Geometry: final body of the model. Coordinates: model frame, mm. Face numbers are marked on the shaded views. A direction names the side the tool comes from. Give positions to 0.01 mm unless a question says otherwise; leave off trailing zeros. Write each loop counter-clockwise with the first axis right and the second up, starting at its lowest first coordinate (ties: lowest second). Pieces come first, ordered by that corner, then holes. Notation, with made-up numbers: (-33.75, 83) -> (-5.75, 83) arc R17 cw to (-5.75, 96) -> close; hole circle Ø2 at (87, 58). An arc over 180 degrees is marked (long way). Answer in a Markdown table with one row per item. Add a question column.
Item 1: First-contact query: P1, Ø1.5, axis at x = 14, z = -6.5, coming from the -Y side; P2, Ø2.5, axis at y = 1.5, z = -5, coming from the -X side; P3, Ø2, axis at x = 4, z = 9, coming from the -Y side. Flat tips, straight axial feed; report the tip coordinate or a pass-through.
Item 2: Material intervals for probe 1 along Z at (x, y) = (0, 8.6); probe 2 along Z at (x, y) = (-10, 9.75); probe 3 along X at (y, z) = (1, -1), sorted ascending. Write a range as from..to.
Item 3: Section query D-D on z = 4. Output: boundary loops of the cut face in (x, y).
Item 4: Draft query along X for the marked faces 1, 2, 3 and 4. Return one class per face: +X half, -X half, draft (parallel to the pull), parting line (faces both ways), or undercut.
Item 5: Section query C-C on x = 0. Output: boundary loops of the cut face in (y, z).
Item 6: Section query B-B on y = 4. Output: boundary loops of the cut face in (x, z).
Item 7: Access query for the marked faces 5, 6 and 7. Directions: +Z, -Z, +X, -X, +Y, -Y. A direction counts if a zero-diameter tool reaches every point of the face in a straight line with its end or side. Return the directions, or none.
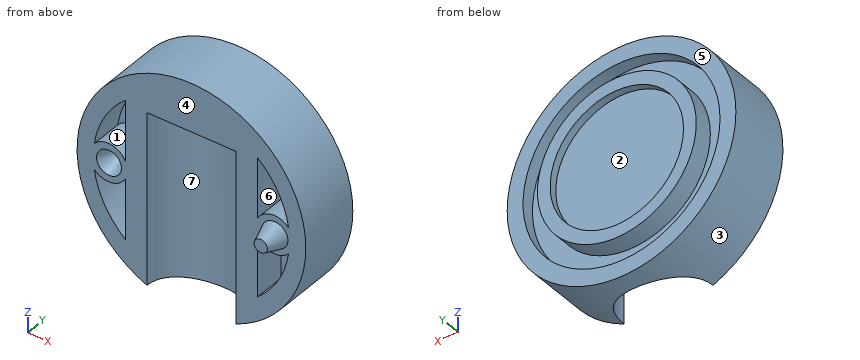
```python
from build123d import *

# Parameters (mm, degrees)
F0_R      = 18
F1_DEPTH  = 10
F2_R      = 15.5
F3_DEPTH  = 2
F5_DEPTH  = 5
F6_R      = 3
F6_R_2    = 1.5
F7_DEPTH  = 5
F8_R      = 12.5
F9_DEPTH  = 3
F10_R     = 10.5
F11_DEPTH = 1.2
F16_W     = 7
F16_H     = 30.015691
F17_ANGLE = -180


with BuildPart() as f1:
    # F0 (on Front) → F1 (new body)
    with BuildSketch(Plane.XZ):
        Circle(F0_R)
    extrude(amount=-F1_DEPTH)

    # F2 (on face) → F3 (cut)
    with BuildSketch(Plane(origin=(0, 10, 0), x_dir=(-1, 0, 0), z_dir=(0, 1, 0))):
        Circle(F2_R)
    extrude(amount=-F3_DEPTH, mode=Mode.SUBTRACT)

    # F4 (on face) → F5 (cut)
    with BuildSketch(Plane.XZ):
        with BuildLine():
            ThreePointArc((10.390717, -10.885251), (15.434695, 0), (10.390717, 10.885251))
            Line((10.390717, 10.885251), (10.390717, -10.885251))
        make_face()
        with BuildLine():
            Line((-10.390717, -10.885251), (-10.390717, 10.885251))
            ThreePointArc((-10.390717, 10.885251), (-15.434695, 0), (-10.390717, -10.885251))
        make_face()
    extrude(amount=-F5_DEPTH, mode=Mode.SUBTRACT)

    # F6 (on face) → F7 (join)
    with BuildSketch(Plane.XZ.offset(-5)):
        with Locations((-13.069113, 0)):
            Circle(F6_R)
        with Locations((13.069113, 0)):
            Circle(F6_R)
        with Locations((13.069113, 0)):
            Circle(F6_R_2, mode=Mode.SUBTRACT)
    extrude(amount=F7_DEPTH)

    # F8 (on face) → F9 (join)
    with BuildSketch(Plane(origin=(0, 8, 0), x_dir=(-1, 0, 0), z_dir=(0, 1, 0))):
        Circle(F8_R)
    extrude(amount=F9_DEPTH)

    # F10 (on face) → F11 (cut)
    with BuildSketch(Plane(origin=(0, 11, 0), x_dir=(-1, 0, 0), z_dir=(0, 1, 0))):
        Circle(F10_R)
    extrude(amount=-F11_DEPTH, mode=Mode.SUBTRACT)

    # F12 (on Top) → F13 (revolve)
    with BuildSketch(Plane.XY):
        Polygon((13.131262, 0), (11.077145, 0), (12.089682, -3), (13.131262, -3), align=None)
    revolve(axis=Axis((13.131262, 2.278473, 0), (0, 1, 0)))

    # F14 (on Top) → F15 (revolve, cut)
    with BuildSketch(Plane.XY):
        Polygon((-13.759153, 2.54694), (-14.932801, 0), (-12.972816, 0), (-12.972816, 2.54694), align=None)
    revolve(axis=Axis((-12.972816, -1.87905, 0), (0, -1, 0)), mode=Mode.SUBTRACT)

    # F16 (on face) → F17 (revolve, cut)
    with BuildSketch(Plane.XZ):
        with Locations((3.5, -4.595023)):
            Rectangle(F16_W, F16_H)
    revolve(axis=Axis((0, 0, -3.36439), (0, 0, -1)), revolution_arc=F17_ANGLE, mode=Mode.SUBTRACT)


solid = f1.part
```
Findings below:
| question | item | result |
|---|---|---|
| 1 | P1 | stops at y = 0 |
| 1 | P2 | stops at x = -17.61 |
| 1 | P3 | stops at y = 4.9 |
| 2 | probe 1 | z = -18..-15.5, -12.5..12.5, 15.5..18 |
| 2 | probe 2 | z = -14.97..-11.84, -7.5..7.5, 11.84..14.97 |
| 2 | probe 3 | x = -17.97..-14.09, -11.86..-6.93, 6.93..11.95, 14.19..17.97 |
| 3 | outline | (-17.55, 0) -> (-14.86, 0) -> (-14.86, 5) -> (-10.39, 5) -> (-10.39, 0) -> (-7, 0) arc R7 cw to (7, 0) -> (10.39, 0) -> (10.39, 5) -> (14.86, 5) -> (14.86, 0) -> (17.55, 0) -> (17.55, 10) -> (14.97, 10) -> (14.97, 8) -> (11.84, 8) -> (11.84, 11) -> (9.71, 11) -> (9.71, 9.8) -> (-9.71, 9.8) -> (-9.71, 11) -> (-11.84, 11) -> (-11.84, 8) -> (-14.97, 8) -> (-14.97, 10) -> (-17.55, 10) -> close |
| 4 | face 1 | undercut |
| 4 | face 2 | undercut |
| 4 | face 3 | parting line |
| 4 | face 4 | draft |
| 5 | outline | (0, 10.41) -> (7, 10.41) -> (7, -18) -> (10, -18) -> (10, -15.5) -> (8, -15.5) -> (8, -12.5) -> (11, -12.5) -> (11, -10.5) -> (9.8, -10.5) -> (9.8, 10.5) -> (11, 10.5) -> (11, 12.5) -> (8, 12.5) -> (8, 15.5) -> (10, 15.5) -> (10, 18) -> (0, 18) -> close |
| 6 | outline | (-5.74, -17.06) -> (-5.74, 10.41) -> (5.74, 10.41) -> (5.74, -17.06) arc R18 ccw (long way) to start; hole (-15.29, -2.01) arc R14.27 ccw to (-10.39, -10.89) -> (-10.39, -1.35) arc R3 cw to start; hole (-15.29, 2.01) arc R3 cw to (-10.39, 1.35) -> (-10.39, 10.89) arc R14.27 ccw to start; hole (10.39, -10.89) arc R14.27 ccw to (15.29, -2.01) arc R3 cw to (10.39, -1.35) -> close; hole (10.39, 1.35) arc R3 cw to (15.29, 2.01) arc R14.27 ccw to (10.39, 10.89) -> close; hole circle Ø3 at (13.07, 0) |
| 7 | face 5 | +Y |
| 7 | face 6 | -Y |
| 7 | face 7 | -Z, -Y |
